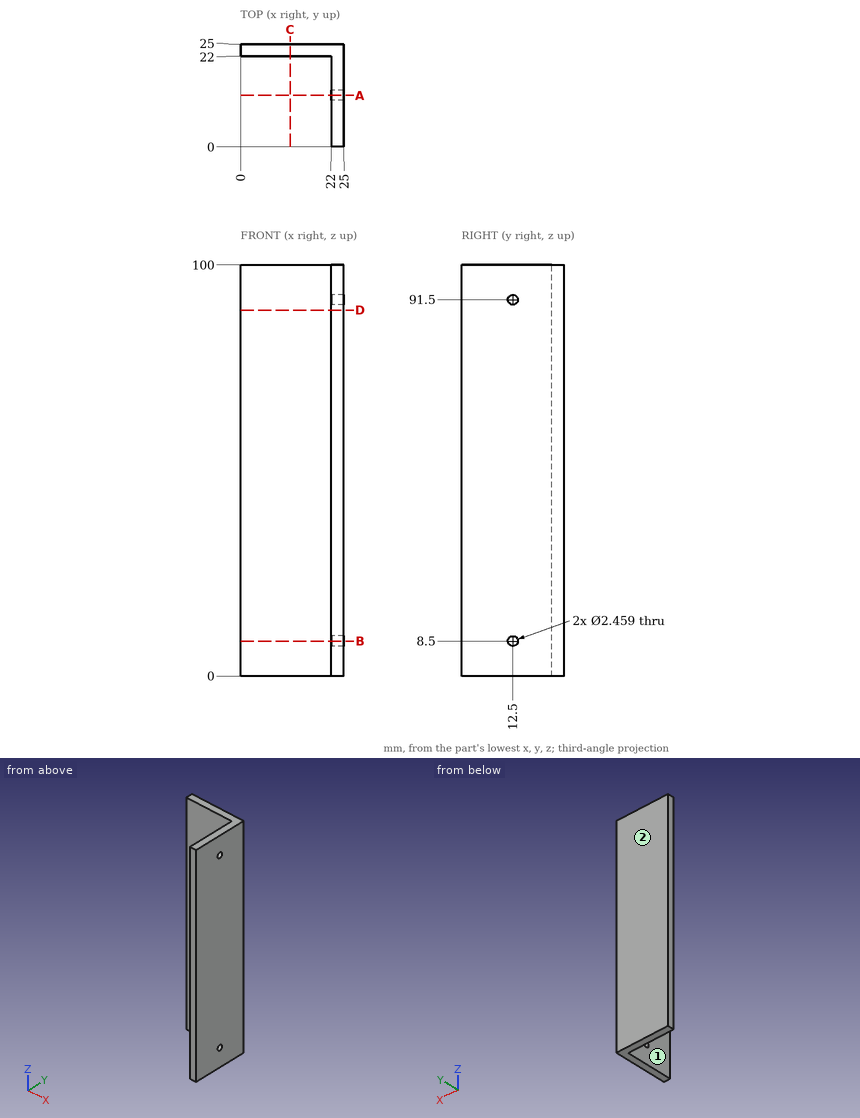
Could you check a few things on this drawing? It's one solid part, dimensions in mm from its lowest x, y, z. A direction names the side the tool comes from. Coordinates: 2 decimals unless noted, no trailing zeros. Order: outer loops, then holes, each group sorted by start corner. A loop starts at its lowest first (then second) coordinate and runs counter-clockwise, first axis right, second up.
1) Imagine slicing it at C-C on x = 12. List the corners of the cut face in (y, z) for me.
2) Imagine slicing it at A-A on y = 12.5. List the corners of the cut face in (x, z) for me, and give its area (3 significant figures).
3) I need wall thicknesses on line 1 (Y direction, x = 23.75, z = 91.5); line 2 (X direction, y = 4, z = 55). Which ranges of each line are inside material? Lowest first, please.
4) Imagine slicing it at B-B on z = 8.5. List the corners of the cut face in (x, y) for me, and give its area (3 significant figures).
5) Will these pins go through, and if not, where does the flat tip stop? pin 1 (2 mm diameter, centred on x = 10.5, z = 54.5, fed in from -Y); pin 2 (1 mm diameter, centred on y = 5.5, z = 61.5, fed in from -X).
6) Which directions (+Z, -Z, +X, -X, +Y, -Y) give clear straight access to the entire face, cutting with the end or side of a thin tool? Please do the marked faces 1 and 2.
7) Imagine slicing it at D-D on z = 89. List the corners of the cut face in (x, y) for me, and give its area (3 significant figures).
Response values:
1. outline: (22, 0) - (25, 0) - (25, 100) - (22, 100) - close
2. outline: (22, 0) - (25, 0) - (25, 7.27) - (22, 7.27) - close; (22, 9.73) - (25, 9.73) - (25, 90.27) - (22, 90.27) - close; (22, 92.73) - (25, 92.73) - (25, 100) - (22, 100) - close
2. area: 285 mm2
3. line 1: y = 0 to 11.27, 13.73 to 25
3. line 2: x = 22 to 25
4. outline: (0, 22) - (22, 22) - (22, 13.73) - (25, 13.73) - (25, 25) - (0, 25) - close; (22, 0) - (25, 0) - (25, 11.27) - (22, 11.27) - close
4. area: 134 mm2
5. pin 1: stops at y = 22
5. pin 2: stops at x = 22
6. face 1: +Z, -Z, -X, -Y
6. face 2: +Z, -Z, +X, -X, +Y
7. outline: (0, 22) - (22, 22) - (22, 0) - (25, 0) - (25, 25) - (0, 25) - close
7. area: 141 mm2
